CAD build for the part. Positions are in the model's coordinates, mm. A direction names the side the tool comes from. Coordinates: 2 decimals unless noted, no trailing zeros. Loops run counter-clockwise (first coordinate to the right, second up) from the corner with the lowest first, then second, coordinate; pieces in that order, holes last. Notation, with made-up numbers: (-36, 13.5) -> (21, 13.5) arc R26 ccw to (21, 36.5) -> close; hole circle Ø1 at (47, -2). An arc over 180 degrees is marked (long way). Write item = value, one per line. Start each with the question number.
(1) Flat gauge pins, fed straight in: P1, Ø3, axis at x = -5.5, y = -16, coming from the +Z side; P2, Ø0.9, axis at x = 20, z = -7, coming from the -Y side; P3, Ø3.5, axis at x = 20, y = 1.5, coming from the +Z side. Where does each tip first touch, or does it go through?
(2) Pull direction Y, two halves, no side cores. Call faces 6 (the face through (-10.45, -15, -13)), 7 (the face through (25.95, 7, -15.56)), 8 (the face through (-18, -30.6, -18)): +Y half, -Y half, draft (parallel to the pull), parting line (faces both ways), or undercut.
(3) Band-saw the part on C-C (z = -18.5). Count the separate pieces of the cut face and the enclosed holes in it, and give its area (3 significant figures).
(4) Drill centre lines: line 1 (Z direction, x = 4, y = -3); line 2 (Y direction, x = 19, z = -12.5); line 3 (Y direction, x = 19, z = -10.5). Where is each one in solid material? Low to high. Write a range as from..to.
(5) Band-saw the part on A-A (y = -19). Write the cut outline in (x, z), and give its area (3 significant figures).
(6) Band-saw the part on B-B (x = 19). Write the cut outline in (y, z).
(7) Tool access for faces 1 (the face through (0, 0, -25)), 2 (the face through (-6.2, -30.2, -21.4)), 3 (the face through (-5.8, -29.5, -21.5)), 4 (the face through (-21, 2, -9)), 5 (the face through (28.194, -28.319, -17.902)): list every direction of +Z, -Z, +X, -X, +Y, -Y with a clear straight run to the whole face (end or side of a thin tool).
```python
from build123d import *

# Parameters (mm, degrees)
PAD017_DEPTH         = 27.5
POCKET043_DEPTH      = 30.601
POCKET044_DEPTH      = 22.501
SKETCH115_W          = 70
SKETCH115_H          = 14
POCKET041_DEPTH      = 30.601
POCKET041_DEPTH_BACK = 30.601
POCKET048_DEPTH      = 9
SKETCH132_R          = 5.5
PAD019_DEPTH         = 5.5
POCKET049_DEPTH      = 180.22267


with BuildPart() as part:
    # Sketch116 → Pad017 (new body)
    with BuildSketch(Plane.XY.offset(2.5)):
        with BuildLine():
            Line((-22.6, 30.6), (22.6, 30.6))
            ThreePointArc((30.6, 22.6), (28.256854, 28.256854), (22.6, 30.6))
            Line((30.6, 22.6), (30.6, -22.6))
            ThreePointArc((22.6, -30.6), (28.256854, -28.256854), (30.6, -22.6))
            Line((22.6, -30.6), (-22.6, -30.6))
            ThreePointArc((-30.6, -22.6), (-28.256854, -28.256854), (-22.6, -30.6))
            Line((-30.6, -22.6), (-30.6, 22.6))
            ThreePointArc((-22.6, 30.6), (-28.256854, 28.256854), (-30.6, 22.6))
        make_face()
    extrude(amount=-PAD017_DEPTH)

    # Sketch117 → Groove014 (revolve, cut)
    with BuildSketch(Plane.XZ.offset(6)):
        Polygon((-26, 3), (-26, -24.2), (-24.4, -8.2), (-23, -6.8), (-23, 3), align=None)
    revolve(axis=Axis((-26, -6, 3), (0, 0, 1)), mode=Mode.SUBTRACT)

    # Sketch118 → Groove013 (revolve, cut)
    with BuildSketch(Plane.XZ.offset(25)):
        Polygon((25, 3), (25, -24.2), (26.6, -8.2), (28, -6.8), (28, 3), align=None)
    revolve(axis=Axis((25, -25, 3), (0, 0, 1)), mode=Mode.SUBTRACT)

    # Sketch119 → Groove016 (revolve, cut)
    with BuildSketch(Plane.XZ.offset(-25)):
        Polygon((25, 3), (25, -24.2), (26.6, -8.2), (28, -6.8), (28, 3), align=None)
    revolve(axis=Axis((25, 25, 3), (0, 0, 1)), mode=Mode.SUBTRACT)

    # Sketch127 → SubtractiveLoft003 section 0
    with BuildSketch(Plane.XY.offset(-22.5)):
        with BuildLine():
            Line((-22.25, 12), (-13.5, 12))
            ThreePointArc((-13.5, 12), (-6, 9.7), (1.5, 12))
            Line((1.5, 12), (10.25, 12))
            Line((10.25, 12), (10.25, -29.5))
            Line((10.25, -29.5), (-22.25, -29.5))
            Line((-22.25, -29.5), (-22.25, 12))
        make_face()
    # Sketch124 → SubtractiveLoft003 section 1
    with BuildSketch(Plane.XY.offset(-16.5)):
        with BuildLine():
            Line((-22.25, 12), (-13.5, 12))
            ThreePointArc((-13.5, 12), (-6, 11.431818), (1.5, 12))
            Line((1.5, 12), (10.25, 12))
            Line((10.25, 12), (10.25, -29.5))
            Line((10.25, -29.5), (-22.25, -29.5))
            Line((-22.25, -29.5), (-22.25, 12))
        make_face()
    loft(mode=Mode.SUBTRACT)

    # Sketch125 → Pocket043 (cut, through all)
    with BuildSketch(Plane.XZ):
        with BuildLine():
            ThreePointArc((-10.45, -19.6), (-9.981371, -20.731371), (-8.85, -21.2))
            Line((-8.85, -21.2), (-3.65, -21.2))
            ThreePointArc((-3.65, -21.2), (-2.518629, -20.731371), (-2.05, -19.6))
            Line((-2.05, 0), (-2.05, -19.6))
            Line((-10.45, 0), (-2.05, 0))
            Line((-10.45, -19.6), (-10.45, 0))
        make_face()
    extrude(amount=POCKET043_DEPTH, mode=Mode.SUBTRACT)

    # SubtractivePipe008: sweep along a path in Sketch126
    with BuildLine(Plane.YZ) as subtractivepipe008_path:
        ThreePointArc((-32.2, -12.527864), (-30.722774, -14.55051), (-30.2, -17))
        Line((-30.2, -17), (-30.2, -23))
        ThreePointArc((-30.2, -23), (-30.722774, -25.44949), (-32.2, -27.472136))
    # Sketch128 → SubtractivePipe008 (sweep, cut)
    with BuildSketch(Plane.XY.offset(-20)):
        with BuildLine():
            ThreePointArc((-11.75, -30.2), (-14.578427, -30.716685), (-17.041503, -32.2))
            Line((-17.041503, -32.2), (4.541503, -32.2))
            ThreePointArc((4.541503, -32.2), (2.078427, -30.716685), (-0.75, -30.2))
            Line((-11.75, -30.2), (-0.75, -30.2))
        make_face()
    sweep(path=subtractivepipe008_path.line, mode=Mode.SUBTRACT)

    # Sketch129 → Pocket044 (cut, through all)
    with BuildSketch(Plane.XY.offset(-20)):
        with BuildLine():
            ThreePointArc((22.834936, 22.25), (23.854356, 21.692811), (25, 21.5))
            ThreePointArc((27, 19.5), (26.414214, 20.914214), (25, 21.5))
            Line((27, 9.5), (27, 19.5))
            ThreePointArc((23.5, 6), (25.974874, 7.025126), (27, 9.5))
            Line((9.5, 6), (23.5, 6))
            ThreePointArc((6, 9.5), (7.025126, 7.025126), (9.5, 6))
            Line((6, 19.5), (6, 9.5))
            ThreePointArc((9.5, 23), (7.025126, 21.974874), (6, 19.5))
            Line((20.669873, 23), (9.5, 23))
            ThreePointArc((22.834936, 22.25), (21.815517, 22.807189), (20.669873, 23))
        make_face()
    extrude(amount=POCKET044_DEPTH, mode=Mode.SUBTRACT)

    # Sketch115 → Pocket041 (cut, two sides)
    with BuildSketch(Plane.XZ) as pocket041_sk:
        with Locations((0, -4)):
            Rectangle(SKETCH115_W, SKETCH115_H)
    extrude(amount=-POCKET041_DEPTH, mode=Mode.SUBTRACT)
    extrude(pocket041_sk.sketch, amount=POCKET041_DEPTH_BACK, mode=Mode.SUBTRACT)

    # Sketch122 → Pocket048 (cut, symmetric)
    with BuildSketch(Plane.XY.offset(-11)):
        Polygon((-26.5, 27), (17.5, 27), (17.5, 23), (15.5, 23), (15.5, 7), (-25.5, 7), (-25.5, 23), (-26.5, 23), align=None)
    extrude(amount=POCKET048_DEPTH, both=True, mode=Mode.SUBTRACT)

    # Sketch132 → Pad019 (join)
    with BuildSketch(Plane.XY.offset(-6)):
        with Locations((19, 0)):
            Circle(SKETCH132_R)
    pad019 = extrude(amount=-PAD019_DEPTH)

    # Sketch121 → Groove017 (revolve, cut)
    with BuildSketch(Plane.XZ):
        Polygon((19, -1.5), (21.8, -1.5), (21.2, -3.148486), (21.2, -13.5), (19, -13.5), align=None)
    groove017 = revolve(axis=Axis((19, 0, -1.5), (0, 0, 1)), mode=Mode.SUBTRACT)

    # Sketch133 → Pocket049 (cut, through all)
    with BuildSketch(Plane.XY.offset(-9)):
        Polygon((23.214657, 0), (21.107328, 3.65), (16.892672, 3.65), (14.785343, 0), (16.892672, -3.65), (21.107328, -3.65), align=None)
    pocket049 = extrude(amount=POCKET049_DEPTH, mode=Mode.SUBTRACT)

    # Mirrored010: Pad019, Groove017, Pocket049 across YZ
    add(pad019.mirror(Plane.YZ))
    add(groove017.mirror(Plane.YZ), mode=Mode.SUBTRACT)
    add(pocket049.mirror(Plane.YZ), mode=Mode.SUBTRACT)


solid = part.part
```
Findings below:
q1.P1 = -22.5
q1.P2 = -5.47
q1.P3 = -9
q2.face_6 = draft
q2.face_7 = undercut
q2.face_8 = -Y half
q3.separate_pieces = 1
q3.enclosed_holes = 3
q3.area = 1,470 mm²
q4.line_1 = -25..-22.5, -16.5..-11
q4.line_2 = -30.6..-2.2, 2.2..6, 23..30.6
q4.line_3 = -5.5..-2.2, 2.2..5.5
q5.outline = (-30.6, -25) -> (30.6, -25) -> (30.6, -11) -> (-2.05, -11) -> (-2.05, -16.5) -> (10.25, -16.5) -> (10.25, -22.5) -> (-22.25, -22.5) -> (-22.25, -16.5) -> (-10.45, -16.5) -> (-10.45, -11) -> (-30.6, -11) -> close
q5.area = 616 mm²
q6.outline = (-30.6, -25) -> (30.6, -25) -> (30.6, -11) -> (23, -11) -> (23, -20) -> (6, -20) -> (6, -11) -> (5.5, -11) -> (5.5, -6) -> (3.65, -6) -> (3.65, -9) -> (2.2, -9) -> (2.2, -13.5) -> (-2.2, -13.5) -> (-2.2, -9) -> (-3.65, -9) -> (-3.65, -6) -> (-5.5, -6) -> (-5.5, -11) -> (-30.6, -11) -> close
q7.face_1 = -Z, +X, -X, +Y, -Y
q7.face_2 = -Y
q7.face_3 = none
q7.face_4 = +Z
q7.face_5 = +Z, -Z, +X, -Y
